from build123d import *

# Parameters (mm, degrees)
SKETCH1_R           = 2.25
SKETCH1_W           = 4.3
SKETCH1_H           = 3
BOSS_EXTRUDE1_DEPTH = 9
SKETCH3_R           = 1.5
BOSS_EXTRUDE2_DEPTH = 4.3
CHAMFER1_SIZE       = 0.5


with BuildPart() as part:
    # Sketch1 → Boss-Extrude1 (new body)
    with BuildSketch(Plane(origin=(0, 0, 0), x_dir=(1, 0, 0), z_dir=(0, 1, 0))):
        with BuildLine():
            Line((-2.15, 4.789572006), (2.15, 4.789572006))
            ThreePointArc((2.15, 4.789572006), (0, -5.25), (-2.15, 4.789572006))
        make_face()
        Circle(SKETCH1_R, mode=Mode.SUBTRACT)
        with Locations((0, 6.289572006)):
            Rectangle(SKETCH1_W, SKETCH1_H)
    extrude(amount=BOSS_EXTRUDE1_DEPTH)

    # Sketch3 → Boss-Extrude2 (add)
    with BuildSketch(Plane(origin=(2.15, 0, 0), x_dir=(0, 0, -1), z_dir=(1, 0, 0))):
        with BuildLine():
            ThreePointArc((12.289572006, 9), (16.789572006, 4.5), (12.289572006, 0))
            Line((12.289572006, 0), (7.789572006, 0))
            Line((7.789572006, 0), (7.789572006, 9))
            Line((7.789572006, 9), (12.289572006, 9))
        make_face()
        with Locations((12.289572006, 4.5)):
            Circle(SKETCH3_R, mode=Mode.SUBTRACT)
    extrude(amount=-BOSS_EXTRUDE2_DEPTH)

    # Chamfer1
    chamfer1_edges = [part.edges().sort_by_distance(p)[0] for p in [
        (0, 9, 5.25),
        (2.15, 9, -8.539572006),
        (2.15, 4.5, -16.789572006),
        (-2.15, 4.5, -16.789572006),
        (-2.15, 9, -8.539572006),
        (-2.15, 0, -8.539572006),
        (2.15, 0, -8.539572006),
        (0, 0, 5.25),
    ]]
    chamfer(chamfer1_edges, length=CHAMFER1_SIZE)


solid = part.part
Input: part model. Units: mm. Frame: model coordinates. A direction names the side the tool comes from. Coordinates: 2 decimals unless noted, no trailing zeros. Loops run counter-clockwise (first coordinate to the right, second up) from the corner with the lowest first, then second, coordinate; pieces in that order, holes last. Notation, with made-up numbers: (-4, 72) -> (13, 72) arc R18 ccw to (13, 97) -> close; hole circle Ø4 at (49, -10.75). An arc over 180 degrees is marked (long way). Write item = value, one per line. Start each with the question number.
Item 1: Cut plane C-C, the plane z = 0. Return loops of the section in (x, y), plus the area to 3 significant figures.
Item 2: Cut plane B-B, the plane y = 4.5. Return loops of the section in (x, z).
Item 3: Cut plane A-A, the plane x = 0. Return loops of the section in (y, z).
Item 4: Mould query, pull axis Z, two halves, no side actions, for faces 1 (the face through (2.15, 4.6, -10.6)), 2 (the face through (2.01, 4.59, -16.43)), 3 (the face through (0.03, 4.95, -13.72)). Classes: pulls with the +Z half, pulls with the -Z half, needs draft (parallel to the pull), parting line crosses it, or undercut.
Item 5: Material intervals for line 1 (Z direction, x = 1.5, y = 5.5); line 2 (X direction, y = 1.5, z = -8.5); line 3 (X direction, y = 1.75, z = 0.75), sorted ascending.
Item 6: Reachability of faces 4 (the face through (-2.15, 4.6, -10.6)), 5 (the face through (0, 9, -4)) from +Z, -Z, +X, -X, +Y, -Y: full face, straight path, thin tool, end or side. Return the list, or none.
Item 7: First-contact query: P1, Ø4, axis at y = 4, z = -8.5, coming from the -X side; P2, Ø2.5, axis at y = 4.5, z = -12.29, coming from the -X side; P3, Ø2.5, axis at y = 5.5, z = -12, coming from the +X side. Flat tips, straight axial feed; report the tip coordinate or a pass-through.
Ans:
q1.outline = (-5.25, 0.5) -> (-4.75, 0) -> (-2.25, 0) -> (-2.25, 9) -> (-4.75, 9) -> (-5.25, 8.5) -> close; (2.25, 0) -> (4.75, 0) -> (5.25, 0.5) -> (5.25, 8.5) -> (4.75, 9) -> (2.25, 9) -> close
q1.area = 53.5 mm²
q2.outline = (-2.15, -16.29) -> (-1.65, -16.79) -> (1.65, -16.79) -> (2.15, -16.29) -> (2.15, -13.79) -> (-2.15, -13.79) -> close; (-2.15, -10.79) -> (2.15, -10.79) -> (2.15, -4.79) arc R5.25 ccw (long way) to (-2.15, -4.79) -> close; hole circle Ø4.5 at (0, 0)
q3.outline = (0, -12.29) arc R4.5 ccw to (9, -12.29) -> (9, -2.25) -> (0, -2.25) -> close; (0, 2.25) -> (9, 2.25) -> (9, 4.75) -> (8.5, 5.25) -> (0.5, 5.25) -> (0, 4.75) -> close; hole circle Ø3 at (4.5, -12.29)
q4.face_1 = needs draft
q4.face_2 = pulls with the -Z half
q4.face_3 = undercut
q5.line_1 = -16.68 to -13.41, -11.17 to -1.68, 1.68 to 5.03
q5.line_2 = -2.15 to 2.15
q5.line_3 = -5.2 to -2.12, 2.12 to 5.2
q6.face_4 = -Z, -X, +Y, -Y
q6.face_5 = +Z, -Z, +X, -X, +Y
q7.P1 = -2.15
q7.P2 = through
q7.P3 = 2.15
